Geometry check sheet. Reference: the model listing, model coordinates, mm. Round coordinates to 2 decimals unless told otherwise and drop trailing zeros. Write each loop counter-clockwise with the first axis right and the second up, starting at its lowest first coordinate (ties: lowest second). Pieces come first, ordered by that corner, then holes. Notation, with made-up numbers: (16.5, 84) - (68.5, 84) arc R33 ccw to (68.5, 112) - close; hole circle Ø8 at (27.25, 5.5). An arc over 180 degrees is marked (long way). Return JSON: item names as keys, results as strings. Group by question number.
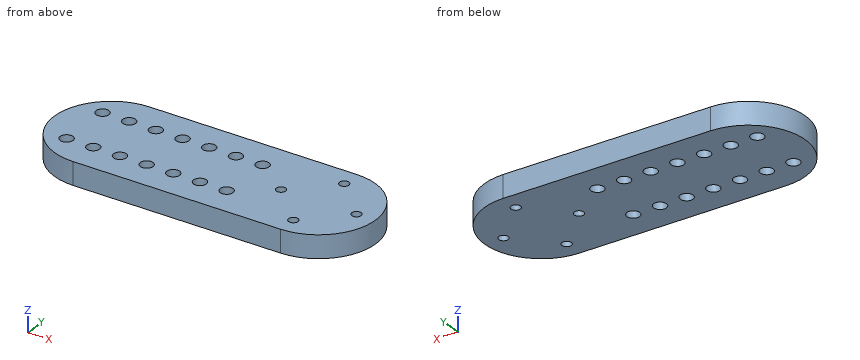
from build123d import *

# Parameters (mm, degrees)
EXTRUDE_1_DEPTH   = 6
M3X0_51_D         = 2.5
HOLE_WIZARD_M31_D = 3.4


with BuildPart() as part:
    # Эскиз1 → Бобышка-Вытянуть1 (new body)
    with BuildSketch(Plane.XY):
        with BuildLine():
            Line((-27.5, 15), (27.5, 15))
            ThreePointArc((27.5, 15), (42.5, 0), (27.5, -15))
            Line((27.5, -15), (-27.5, -15))
            ThreePointArc((-27.5, -15), (-42.5, 0), (-27.5, 15))
        make_face()
    extrude(amount=EXTRUDE_1_DEPTH)

    # Отверстие обработанное метчиком M3x0.51 (through all)
    with Locations(Plane.XY.offset(6)):
        with Locations((27.5, 10), (37.5, 0), (27.5, -10), (17.5, 0)):
            Hole(M3X0_51_D / 2)

    # Отверстие с зазором M31 (through all)
    with Locations(Plane.XY.offset(6)):
        with Locations((-34.571067812, 7.071067812), (-20.428932188, 7.071067812), (-6.286796564, 7.071067812), (7.855339059, 7.071067812), (7.855339059, -7.071067812), (-6.286796564, -7.071067812), (-20.428932188, -7.071067812), (-34.571067812, -7.071067812), (-27.5, -7.071067812), (-27.5, 7.071067812), (-13.357864376, 7.071067812), (-13.357864376, -7.071067812), (0.784271247, -7.071067812), (0.784271247, 7.071067812)):
            Hole(HOLE_WIZARD_M31_D / 2)


solid = part.part
1. Section check C-C (y = -10). Enter the section's corners in (x, z).
2. Depth check by flat-ended pin: pin 1 Ø1 at (y, z) = (-10, 2) entering from +X; pin 2 Ø1.5 at (y, z) = (-1.5, 3.5) entering from -X. Enter the tip coordinate at first touch or a pass-through.
3. Section check B-B (x = 17.5). Enter the section's corners in (y, z), and give its area (3 significant figures).
4. Material ranges on line 1 along Y through (x, z) = (-27.5, 4.4); line 2 along Y through (x, z) = (-35, 1.05); line 3 along X through (y, z) = (1, 1.45), recorded low to high.
5. Section check A-A (y = 0). Enter the section's corners in (x, z), and give its area (3 significant figures).
6. Section check D-D (z = 3.7). State how many separate pieces and enclosed holes the cut face has, and give its area (3 significant figures).
Result sheet:
{
 "1": {"outline": "(-38.68, 0) - (26.25, 0) - (26.25, 6) - (-38.68, 6) - close; (28.75, 0) - (38.68, 0) - (38.68, 6) - (28.75, 6) - close"},
 "2": {"pin 1": "stops at x = 39.11", "pin 2": "stops at x = -42.48"},
 "3": {"outline": "(-15, 0) - (-1.25, 0) - (-1.25, 6) - (-15, 6) - close; (1.25, 0) - (15, 0) - (15, 6) - (1.25, 6) - close", "area": "165 mm²"},
 "4": {"line 1": "y = -15 to -8.77, -5.37 to 5.37, 8.77 to 15", "line 2": "y = -12.99 to -8.72, -5.43 to 5.43, 8.72 to 12.99", "line 3": "x = -42.47 to 16.75, 18.25 to 36.75, 38.25 to 42.47"},
 "5": {"outline": "(-42.5, 0) - (16.25, 0) - (16.25, 6) - (-42.5, 6) - close; (18.75, 0) - (36.25, 0) - (36.25, 6) - (18.75, 6) - close; (38.75, 0) - (42.5, 0) - (42.5, 6) - (38.75, 6) - close", "area": "480 mm²"},
 "6": {"separate pieces": "1", "enclosed holes": "18", "area": "2,210 mm²"}
}
